```python
from build123d import *

# Parameters (mm, degrees)
EXTRUDE_1_DEPTH     = 177.8
SKETCH_2_R          = 1.5875
CUT_EXTRUDE_1_DEPTH = 254


with BuildPart() as part:
    # 스케치1 → 보스-돌출1 (new body)
    with BuildSketch(Plane.XY):
        Polygon((-34.442078201, -34.169098619), (-21.742078201, -56.166143875), (-10.743555573, -62.516143875), (-9.949805573, -61.141328546), (-20.579947544, -55.004013218), (-32.854578201, -33.743729276), (-32.854578201, 67.430901381), (-34.442078201, 67.430901381), align=None)
    extrude(amount=EXTRUDE_1_DEPTH)

    # 스케치2 → 컷-돌출1 (cut)
    with BuildSketch(Plane.ZY.offset(34.442078201)):
        with Locations((158.75, 48.380901381)):
            Circle(SKETCH_2_R)
        with Locations((88.9, 48.380901381)):
            Circle(SKETCH_2_R)
        with Locations((19.05, 48.380901381)):
            Circle(SKETCH_2_R)
    extrude(amount=-CUT_EXTRUDE_1_DEPTH, mode=Mode.SUBTRACT)


solid = part.part
```
The model under review builds one solid part; all positions refer to its coordinate system, in mm. A direction names the side the tool comes from. Coordinates: 2 decimals unless noted, no trailing zeros. Loops run counter-clockwise (first coordinate to the right, second up) from the corner with the lowest first, then second, coordinate; pieces in that order, holes last. Notation, with made-up numbers: (-1.5, -24.75) -> (3.5, -24.75) arc R30 cw to (3.5, 8.25) -> close; hole circle Ø1 at (83.25, 26). An arc over 180 degrees is marked (long way). Answer as CSV lines item,"result".
Item 1: Machinability: for faces 1 (the flat face through (-32.855, 16, 88)), 2 (the flat face through (-16.32, -59.297, 87.655)), which of the approach directions +Z, -Z, +X, -X, +Y, -Y give a long, thin tool a straight path to every point of the face, cutting with its end or side? Answer none if there is none.
Results below:
face 1,"+Z, -Z, +X, +Y"
face 2,"+Z, -Z, -X, -Y"
Item 2: For L1, parallel to X at y = -16, z = 49; L2, parallel to Y at x = -33.2, z = 88.9; L3, parallel to Y at x = -33.8, z = 19.05, list the stretches that pass through material, from the lowest coordinate up.
Results below:
L1,"x = -34.44 to -32.85"
L2,"y = -36.32 to 46.79, 49.97 to 67.43"
L3,"y = -35.28 to 46.79, 49.97 to 67.43"
Item 3: Take a section at C-C, the plane x = -18.75. State the section outline as (y, z) points, and give its area (3 significant figures).
Results below:
outline,"(-57.89, 0) -> (-56.06, 0) -> (-56.06, 177.8) -> (-57.89, 177.8) -> close"
area,"326 mm2"
Item 4: Take a section at B-B, the plane y = 20.5. State the section outline as (x, z) points.
Results below:
outline,"(-34.44, 0) -> (-32.85, 0) -> (-32.85, 177.8) -> (-34.44, 177.8) -> close"
Item 5: Insertion check: pin 1 (8 mm diameter, centred on x = -25.5, z = 141.5, fed in from -Y); pin 2 (1.9 mm diameter, centred on y = 48.38, z = 88.9, fed in from +X); pin 3 (1.5 mm diameter, centred on y = 52.5, z = 108, fed in from +X); pin 4 (5 mm diameter, centred on x = -12.5, z = 143, fed in from +Y). Each pin has a flat end and moves straight along its axis. Give the tip position at first contact, or say it passes through.
Results below:
pin 1,"stops at y = -56.31"
pin 2,"passes through"
pin 3,"stops at x = -32.85"
pin 4,"stops at y = -58.23"
Item 6: Take a section at A-A, the plane z = 29. State the section outline as (x, y) points, and give its area (3 significant figures).
Results below:
outline,"(-34.44, -34.17) -> (-21.74, -56.17) -> (-10.74, -62.52) -> (-9.95, -61.14) -> (-20.58, -55) -> (-32.85, -33.74) -> (-32.85, 67.43) -> (-34.44, 67.43) -> close"
area,"220 mm2"
